from build123d import *

# Parameters (mm, degrees)
SKETCH1_R               = 10.95
SKETCH1_R_2             = 6.05
BOSS_EXTRUDE1_DEPTH     = 2
BOSS_EXTRUDE2_START     = 12
SKETCH1_3_R             = 10.95
SKETCH1_3_R_2           = 6.05
BOSS_EXTRUDE2_DEPTH     = 12
BOSS_EXTRUDE3_START     = -2.5
SKETCH2_R               = 12.95
SKETCH2_R_2             = 10.95
BOSS_EXTRUDE3_DEPTH     = 11.5
CUT_EXTRUDE1_DEPTH      = 22.895319134
CUT_EXTRUDE1_DEPTH_BACK = 22.895319134
SKETCH3_W               = 100
SKETCH3_H               = 24
CUT_EXTRUDE3_DEPTH      = 22.347189511
CUT_EXTRUDE3_DEPTH_BACK = 22.347189511
SKETCH5_W               = 18
SKETCH5_H               = 4
CUT_EXTRUDE4_DEPTH      = 22.347189511
FILLET1_R               = 2
CUT_EXTRUDE5_DEPTH      = 22.347189684
CUT_EXTRUDE5_DEPTH_BACK = 22.347189684
SKETCH6_R               = 1.6


with BuildPart() as part:
    # Sketch1 → Boss-Extrude1 (new body)
    # profile 1 of 2: a face of its own
    with BuildSketch(Plane(origin=(0, 0, 0), x_dir=(1, 0, 0), z_dir=(0, 1, 0))):
        with Locations(Location((0, 0, 0), (0, 0, 270))):
            Circle(SKETCH1_R)
        Circle(SKETCH1_R_2, mode=Mode.SUBTRACT)
    # profile 2 of 2: a face of its own
    with BuildSketch(Plane(origin=(0, 0, 0), x_dir=(1, 0, 0), z_dir=(0, 1, 0))):
        Circle(SKETCH1_R_2)
    extrude(amount=-BOSS_EXTRUDE1_DEPTH)

    # Sketch1<3> → Boss-Extrude2 (add)
    with BuildSketch(Plane(origin=(0, 0, 0), x_dir=(1, 0, 0), z_dir=(0, 1, 0)).offset(BOSS_EXTRUDE2_START)):
        with Locations(Location((0, 0, 0), (0, 0, 270))):
            Circle(SKETCH1_3_R)
        with Locations(Location((0, 0, 0), (0, 0, 270))):
            Circle(SKETCH1_3_R_2, mode=Mode.SUBTRACT)
    extrude(amount=-BOSS_EXTRUDE2_DEPTH)

    # Sketch2 → Boss-Extrude3 (add)
    with BuildSketch(Plane(origin=(0, 12, 0), x_dir=(1, 0, 0), z_dir=(0, 1, 0)).offset(BOSS_EXTRUDE3_START)):
        with Locations(Location((0, 0, 0), (0, 0, 270))):
            Circle(SKETCH2_R)
        with Locations(Location((0, 0, 0), (0, 0, 270))):
            Circle(SKETCH2_R_2, mode=Mode.SUBTRACT)
    extrude(amount=-BOSS_EXTRUDE3_DEPTH)

    # Sketch3 → Cut-Extrude1 (cut, two sides: drawn at the far end of the back side and taken through both)
    with BuildSketch(Plane(origin=(0, 0, 0), x_dir=(1, 0, 0), z_dir=(0, 1, 0)).offset(-CUT_EXTRUDE1_DEPTH_BACK)):
        with Locations((0, -24)):
            Rectangle(SKETCH3_W, SKETCH3_H)
        with Locations((0, 24)):
            Rectangle(SKETCH3_W, SKETCH3_H)
    extrude(amount=CUT_EXTRUDE1_DEPTH + CUT_EXTRUDE1_DEPTH_BACK, mode=Mode.SUBTRACT)

    # Sketch4 → Cut-Extrude3 (cut, two sides: drawn at the far end of the back side and taken through both)
    with BuildSketch(Plane.XY.offset(-CUT_EXTRUDE3_DEPTH_BACK)):
        Polygon((13, 15), (5, 15), (13, 7), align=None)
    extrude(amount=CUT_EXTRUDE3_DEPTH + CUT_EXTRUDE3_DEPTH_BACK, mode=Mode.SUBTRACT)

    # Sketch5 → Cut-Extrude4 (cut, through all)
    with BuildSketch(Plane(origin=(0, 0, 0), x_dir=(1, 0, 0), z_dir=(0, 1, 0))):
        with Locations((-11, 0)):
            Rectangle(SKETCH5_W, SKETCH5_H)
    extrude(amount=CUT_EXTRUDE4_DEPTH, mode=Mode.SUBTRACT)

    # Fillet1
    fillet1_edges = [part.edges().sort_by_distance(p)[0] for p in [
        (-8.237831116, 12, 2),
        (-8.237831116, 12, -2),
        (-9.252243836, 0, -2),
        (-9.252243836, 0, 2),
    ]]
    fillet(fillet1_edges, radius=FILLET1_R - 0.0001)  # a hair under: the kernel refuses the full size

    # Sketch6 → Cut-Extrude5 (cut, two sides: drawn at the far end of the back side and taken through both)
    with BuildSketch(Plane(origin=(0, 0, 0), x_dir=(1, 0, 0), z_dir=(0, 1, 0)).offset(-CUT_EXTRUDE5_DEPTH_BACK)):
        with Locations(Location((0, 0, 0), (0, 0, 270))):
            Circle(SKETCH6_R)
    extrude(amount=CUT_EXTRUDE5_DEPTH + CUT_EXTRUDE5_DEPTH_BACK, mode=Mode.SUBTRACT)


solid = part.part
The listing builds one solid part. Answer for the finished solid, in the listing's coordinates (mm). A direction names the side the tool comes from. Round coordinates to 2 decimals unless told otherwise and drop trailing zeros. Write each loop counter-clockwise with the first axis right and the second up, starting at its lowest first coordinate (ties: lowest second). Pieces come first, ordered by that corner, then holes. Notation, with made-up numbers: (26.25, -24) - (48.25, -24) arc R14 cw to (48.25, -7) - close; hole circle Ø3 at (14, 40). An arc over 180 degrees is marked (long way). Use a Markdown table: item, result. Add a question column.
1. The part is cut by section C-C (z = 0.75). Write down the section's boundary in (x, y).
2. The part is cut by section B-B (y = 4.5). Write down the section's boundary in (x, z).
3. For a pull along Y with two mould halves and no side action, classify faces 6 (the face through (0, 4, 12)), 7 (the face through (0, -2, 2)), 8 (the face through (-1.5, 0, 1.3)) as +Y half, -Y half, draft (parallel to the pull), parting line (faces both ways), or undercut.
4. A tool of negligible diameter and unlimited length cuts with its end or side. For faces 1 (the face through (5, 12, 5)), 2 (the face through (6.044, 6.084, 0.266)), 3 (the face through (-3, 9.5, 11)), 4 (the face through (-0.365, 10.767, -10.944)), 5 (the face through (-9.28, 0.6, 1.43)), from which of +Z, -Z, +X, -X, +Y, -Y can it reach the whole face along a straight path? Write none if from no direction.
5. The part is cut by section D-D (z = -9). Write down the section's boundary in (x, y), and give its area (3 significant figures).
6. Consider line 1 (Z direction, x = 0, y = 4.5); line 2 (Z direction, x = 0, y = -0.85); line 3 (X direction, y = -0.6, z = 0). Determine where each line is inside the solid, lowest interval first.
7. Flat-ended cylindrical pins translate along their axes: P1, Ø5.5, axis at x = -11, y = 6.5, coming from the +Z side; P2, Ø3, axis at x = -7, y = 3, coming from the +Z side; P3, Ø4, axis at y = 8.5, z = -2, coming from the -X side. Find the tip coordinate at first contact, or state that the pin passes through.
8. The part is cut by section A-A (x = 0). Write down the section's boundary in (y, z), and give its area (3 significant figures).
Reported:
| question | item | result |
|---|---|---|
| 1 | outline | (-12.93, -2) - (-1.41, -2) - (-1.41, 0) - (-6, 0) - (-6, 0.15) - (-12.93, 0.15) - close; (1.41, -2) - (12.93, -2) - (12.93, 7.07) - (8, 12) - (6, 12) - (6, 0) - (1.41, 0) - close |
| 2 | outline | (-12.79, -2) arc R12.95 ccw to (-4.87, -12) - (4.87, -12) arc R12.95 ccw to (4.87, 12) - (-4.87, 12) arc R12.95 ccw to (-12.79, 2) - (-5.71, 2) arc R6.05 cw (long way) to (-5.71, -2) - close |
| 3 | face 6 | draft |
| 3 | face 7 | -Y half |
| 3 | face 8 | +Y half |
| 4 | face 1 | +Z, -Z, +X, -X, +Y |
| 4 | face 2 | +Y |
| 4 | face 3 | +Z, +Y |
| 4 | face 4 | -Z, +Y |
| 4 | face 5 | -X, +Y |
| 5 | outline | (-9.31, -2) - (9.31, -2) - (9.31, 9.5) - (6.24, 9.5) - (6.24, 12) - (-6.24, 12) - (-6.24, 9.5) - (-9.31, 9.5) - close |
| 5 | area | 245 mm^2 |
| 6 | line 1 | -12 to -6.05, 6.05 to 12 |
| 6 | line 2 | -12 to -1.6, 1.6 to 12 |
| 6 | line 3 | -12.95 to -1.6, 1.6 to 12.95 |
| 7 | P1 | z = 9.98 |
| 7 | P2 | z = 11.72 |
| 7 | P3 | x = -12.79 |
| 8 | outline | (-2, -12) - (9.5, -12) - (9.5, -10.95) - (12, -10.95) - (12, -6.05) - (0, -6.05) - (0, -1.6) - (-2, -1.6) - close; (-2, 1.6) - (0, 1.6) - (0, 6.05) - (12, 6.05) - (12, 10.95) - (9.5, 10.95) - (9.5, 12) - (-2, 12) - close |
| 8 | area | 179 mm^2 |
